Can you work these out from the model? Positions are in its coordinate system, mm. Face numbers are marked on the shaded views. A direction names the side the tool comes from. Coordinates: 2 decimals unless noted, no trailing zeros. Loops run counter-clockwise (first coordinate to the right, second up) from the corner with the lowest first, then second, coordinate; pieces in that order, holes last.
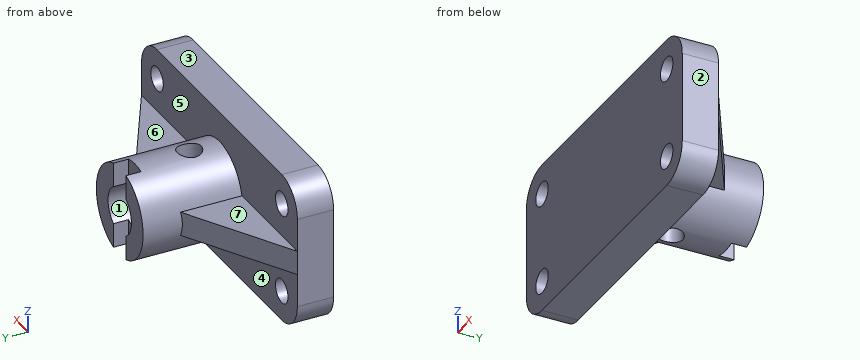
```python
from build123d import *

# Parameters (mm, degrees)
SKETCH_1_R          = 4
EXTRUDE_1_DEPTH     = 12
SKETCH_2_R          = 15
SKETCH_2_R_2        = 7.5
EXTRUDE_2_DEPTH     = 33
SKETCH_3_R          = 4
SKETCH_3_W          = 8
SKETCH_3_H          = 5
CUT_EXTRUDE_1_DEPTH = 84.815273071
RIB_1_REACH         = 73.764
SKETCH_4_WALL_W     = 185.83828981
SKETCH_4_WALL_H     = 8


with BuildPart() as part:
    # 草图1 → 凸台-拉伸1 (new body)
    with BuildSketch(Plane(origin=(0, 0, 0), x_dir=(1, 0, 0), z_dir=(0, 1, 0))):
        with BuildLine():
            Line((-40, -25), (40, -25))
            ThreePointArc((40, -25), (47.071067812, -22.071067812), (50, -15))
            Line((50, -15), (50, 15))
            ThreePointArc((50, 15), (47.071067812, 22.071067812), (40, 25))
            Line((40, 25), (-40, 25))
            ThreePointArc((-40, 25), (-47.071067812, 22.071067812), (-50, 15))
            Line((-50, 15), (-50, -15))
            ThreePointArc((-50, -15), (-47.071067812, -22.071067812), (-40, -25))
        make_face()
        with Locations(Location((-40, 15, 0), (0, 0, 270))):
            Circle(SKETCH_1_R, mode=Mode.SUBTRACT)
        with Locations(Location((-40, -15, 0), (0, 0, 270))):
            Circle(SKETCH_1_R, mode=Mode.SUBTRACT)
        with Locations(Location((40, -15, 0), (0, 0, 270))):
            Circle(SKETCH_1_R, mode=Mode.SUBTRACT)
        with Locations(Location((40, 15, 0), (0, 0, 270))):
            Circle(SKETCH_1_R, mode=Mode.SUBTRACT)
    extrude(amount=EXTRUDE_1_DEPTH)

    # 草图2 → 凸台-拉伸2 (add)
    with BuildSketch(Plane(origin=(0, 12, 0), x_dir=(1, 0, 0), z_dir=(0, 1, 0))):
        with Locations(Location((0, 0, 0), (0, 0, 90))):
            Circle(SKETCH_2_R)
        with Locations(Location((0, 0, 0), (0, 0, 270))):
            Circle(SKETCH_2_R_2, mode=Mode.SUBTRACT)
    extrude(amount=EXTRUDE_2_DEPTH)

    # 草图3 → 切除-拉伸1 (cut, through all)
    with BuildSketch(Plane.XY.offset(25)):
        with Locations((0, 22)):
            Circle(SKETCH_3_R)
        with Locations((0, 42.5)):
            Rectangle(SKETCH_3_W, SKETCH_3_H)
    extrude(amount=-CUT_EXTRUDE_1_DEPTH, mode=Mode.SUBTRACT)

    # 草图4 wall → 筋1 (add, up to next)
    with BuildSketch(Plane(origin=(-32.5, 22, 0), x_dir=(0.868243142124, 0.496138938357, 0), z_dir=(-0.496138938357, 0.868243142124, 0)), mode=Mode.PRIVATE) as rib_1_sk1:
        Rectangle(SKETCH_4_WALL_W, SKETCH_4_WALL_H)
    rib_1_tool1 = extrude(rib_1_sk1.sketch, amount=-RIB_1_REACH, mode=Mode.PRIVATE) - part.part
    rib_1 = rib_1_tool1.solids().sort_by_distance((-32.5, 22, 0))[0]
    add(rib_1)

    # 镜向1: 筋1 across plane
    add(rib_1.mirror(Plane(origin=(0, 0, 0), x_dir=(0, 0, 1), z_dir=(1, 0, 0))))


solid = part.part
```
Item 1: Suppose I cut it at C-C, the plane y = 22. Please give me the cut outline in (x, z), plus the area to 3 significant figures.
Results are:
outline: (-32.5, -4) - (-14.46, -4) arc R15 ccw to (-4, -14.46) - (-4, -6.34) arc R7.5 cw to (-4, 6.34) - (-4, 14.46) arc R15 ccw to (-14.46, 4) - (-32.5, 4) - close; (4, -14.46) arc R15 ccw to (14.46, -4) - (32.5, -4) - (32.5, 4) - (14.46, 4) arc R15 ccw to (4, 14.46) - (4, 6.34) arc R7.5 cw to (4, -6.34) - close
area: 690 mm2
Item 2: Suppose I cut it at D-D, the plane z = 13. Please give me the cut outline in (x, y), plus the area to 3 significant figures.
Results are:
outline: (-50, 0) - (-43.46, 0) - (-43.46, 12) - (-50, 12) - close; (-36.54, 0) - (36.54, 0) - (36.54, 12) - (7.48, 12) - (7.48, 45) - (4, 45) - (4, 40) - (-4, 40) - (-4, 45) - (-7.48, 45) - (-7.48, 12) - (-36.54, 12) - close; (43.46, 0) - (50, 0) - (50, 12) - (43.46, 12) - close; hole circle Ø8 at (0, 22)
area: 1,440 mm2
Item 3: On a 3-axis mill with a long thin cutter (end or side, diameter ignored), from which of +Z, -Z, +X, -X, +Y, -Y can I reach the whole of each face in a straight line? I mean the marked faces 4, 5, 6 and 7. Say none if no direction works.
Results are:
face 4: -Z, +Y
face 5: +Z, +Y
face 6: +Z, +X, +Y
face 7: +Z, -X, +Y
Item 4: Suppose I cut it at B-B, the plane z = 0. Please give me the cut outline in (x, y), plus the area to 4 significant figures.
Results are:
outline: (-50, 0) - (50, 0) - (50, 12) - (15, 32) - (15, 45) - (7.5, 45) - (7.5, 12) - (-7.5, 12) - (-7.5, 45) - (-15, 45) - (-15, 32) - (-50, 12) - close
area: 2,395 mm2
Item 5: I'm going to push flat-ended pins straight in: P1, Ø5.5, axis at y = 43, z = 11, coming from the -X side; P2, Ø2.5, axis at y = 43, z = -11.5, coming from the +X side; P3, Ø16, axis at x = 38, y = 21, coming from the +Z side; P4, Ø6, axis at x = -40.5, y = 21, coming from the -Z side. Where does each tip first touch, or does it pass through?
Results are:
P1: stops at x = -12.53
P2: stops at x = 10.95
P3: stops at z = 4
P4: passes through
Item 6: We'd pull the mould along Z, two halves only. Please class the marked faces 1, 2 and 3: +Z half, -Z half, draft (parallel to the pull), parting line (faces both ways), or undercut.
Results are:
face 1: undercut
face 2: draft
face 3: +Z half
Item 7: I need wall thicknesses on line 1 along X through (y, z) = (5, -15); line 2 along Y through (x, z) = (0, 9.25); line 3 along Z through (x, y) = (4, 31). Which ranges of each line are inside material? Lowest first, please.
Results are:
line 1: x = -50 to -44, -36 to 36, 44 to 50
line 2: y = 0 to 18, 26 to 40
line 3: z = -14.46 to -6.34, 6.34 to 14.46
Item 8: Suppose I cut it at A-A, the plane y = 14. Please give me the cut outline in (x, z), plus the area to 3 significant figures.
Results are:
outline: (-46.5, -4) - (-14.46, -4) arc R15 ccw to (14.46, -4) - (46.5, -4) - (46.5, 4) - (14.46, 4) arc R15 ccw to (-14.46, 4) - (-46.5, 4) - close; hole circle Ø15 at (0, 0)
area: 1,040 mm2
